Can you work these out from the model? Positions are in its coordinate system, mm. A direction names the side the tool comes from. Coordinates: 2 decimals unless noted, no trailing zeros. Order: outer loops, then holes, each group sorted by start corner. A loop starts at its lowest first (then second) coordinate and runs counter-clockwise, first axis right, second up. Notation, with made-up numbers: (-31, 12.25) -> (-14, 12.25) arc R19 ccw to (-14, 21.25) -> close; hole circle Ø11 at (-29.5, 78.5). An arc over 180 degrees is marked (long way). Answer in a Markdown table with one row per item. Add a question column.
1. If I drill on line 1 along X through (y, z) = (-0.5, -45.5); line 2 along Z through (x, y) = (-8.75, 8); line 3 along Y through (x, z) = (-2.5, -3), over which ranges is the centre line in solid material (lowest first)? Write a range as [from, to].
2. Will these pins go through, and if not, where does the flat tip stop? pin 1 (10 mm diameter, centred on x = 6.5, z = -44, fed in from -Y); pin 2 (6 mm diameter, centred on x = 3.5, z = -83.5, fed in from -Y); pin 3 (5 mm diameter, centred on y = 5.5, z = -69.5, fed in from +X).
3. Imagine slicing it at C-C on x = 11.5. Write out the boundary of the cut face in (y, z).
4. Imagine slicing it at B-B on z = -77.5. Write out the boundary of the cut face in (x, y), plus the area to 3 significant figures.
5. On a 3-axis mill with a long thin cutter (end or side, diameter ignored), from which of +Z, -Z, +X, -X, +Y, -Y can I reach the whole of each face in a straight line? I mean faces 4 (the face through (-1.04, -7.93, -80.66)), 5 (the face through (10.44, 5.92, 5.23)). Say none if no direction works.
6. We'd pull the mould along X, two halves only. Please class faces 1 (the face through (0, 12, 5)), 2 (the face through (-10.44, -5.92, 5.23)), 3 (the face through (-1.73, -7.81, -30.57)): pulls with the +X half, pulls with the -X half, needs draft (parallel to the pull), parting line crosses it, or undercut.
7. Imagine slicing it at D-D on x = -11.75. Write out the boundary of the cut face in (y, z), plus the area to 3 significant figures.
Solid Edge part; units mm, degrees
sketch "Sketch1" plane through (0, 0, 0) normal (0, 0, 1) x (1, 0, 0)
  circle A0 centre (0, 0) radius 13.92
extrude "Protrusion1" add sketch "Sketch1" along normal blind 10.32
sketch "Sketch2" plane through (0, 0, 0) normal (0, 0, -1) x (1, 0, 0)
  circle A0 centre (0, 0) radius 8
extrude "Protrusion2" add sketch "Sketch2" along normal blind 100
sketch "Sketch3" plane through (0, 0, -100) normal (0, 0, -1) x (1, 0, 0)
  circle A0 centre (0, 0) radius 7.9997
extrude "Cutout1" cut sketch "Sketch3" against normal blind 38 flip side to cut
chamfer "Chamfer_1" distance 1.2 angle 45 1 edges at (-7.9997, 0, -100)
sketch "Sketch4" plane through (0, 0, 10.32) normal (0, 0, 1) x (1, 0, 0)
  line L0 (-7.0545, 12) -> (7.0545, 12)
extrude "Cutout2" cut sketch "Sketch4" against normal up to next material side at (0, 12.05, 10.32)
pattern_circular "Pattern1" count 6 over 360 about axis through (0, 0, 10.32) along (0, 0, 1) of "Cutout2"
properties part number "118588" material "Stainless Steel, 304"
Answers follow:
| question | item | result |
|---|---|---|
| 1 | line 1 | x = [-7.98, 7.98] |
| 1 | line 2 | z = [0, 10.32] |
| 1 | line 3 | y = [-7.6, 7.6] |
| 2 | pin 1 | stops at y = -7.86 |
| 2 | pin 2 | stops at y = -7.98 |
| 2 | pin 3 | stops at x = 7.42 |
| 3 | outline | (-4.08, 0) -> (4.08, 0) -> (4.08, 10.32) -> (-4.08, 10.32) -> close |
| 4 | outline | circle Ø16 at (0, 0) |
| 4 | area | 201 mm² |
| 5 | face 4 | -Z |
| 5 | face 5 | +Z, -Z, +X, +Y |
| 6 | face 1 | needs draft |
| 6 | face 2 | pulls with the -X half |
| 6 | face 3 | parting line crosses it |
| 7 | outline | (-3.65, 0) -> (3.65, 0) -> (3.65, 10.32) -> (-3.65, 10.32) -> close |
| 7 | area | 75.3 mm² |
